Autodesk Inventor part; units mm, degrees
ref_plane "YZ Plane" through (0, 0, 0) normal (1, 0, 0) x (0, 1, 0)
ref_plane "XZ Plane" through (0, 0, 0) normal (0, 1, 0) x (-1, 0, 0)
ref_plane "XY Plane" through (0, 0, 0) normal (0, 0, 1) x (1, 0, 0)
sketch "Sketch2" plane through (0, 0, 0) normal (0, 0, 1) x (1, 0, 0)
  line L0 (0, 12.7) -> (3.6703, 12.7)
  line L1 (0, 12.7) -> (-3.6703, 12.7)
  line L2 (0, 0) -> (3.6703, 0)
  line L3 (0, 0) -> (-3.6703, 0)
  line L4 (-3.6703, 0) -> (-7.3406, 6.35)
  line L5 (-7.3406, 6.35) -> (-3.6703, 12.7)
  line L6 (3.6703, 12.7) -> (7.3406, 6.35)
  line L7 (7.3406, 6.35) -> (3.6703, 0)
  line L8 (0, 0) -> (0, 6.35)
  circle A0 centre (0, 6.35) radius 8.255
  dimension "d11" = 6.35
  dimension "d12" = 16.51
extrude "Extrusion2" add sketch "Sketch2" along normal blind 6.223
sketch "Sketch3" plane through (0, 6.35, 6.223) normal (0, 0, 1) x (1, 0, 0)
  line L0 (-3.6703, -6.35) -> (-7.3406, 0)
  line L1 (-7.3406, 0) -> (-3.6703, 6.35)
  line L2 (-3.6703, 6.35) -> (3.6703, 6.35)
  line L3 (3.6703, 6.35) -> (7.3406, 0)
  line L4 (7.3406, 0) -> (3.6703, -6.35)
  line L5 (3.6703, -6.35) -> (-3.6703, -6.35)
  circle A0 centre (0, 0) radius 8.255
  point P0 (0, -6.35)
extrude "Extrusion3" add sketch "Sketch3" along normal blind 3.302
sketch "Sketch4" plane through (0, 6.35, 9.525) normal (0, 0, 1) x (1, 0, 0)
  line L0 (-7.3406, 0) -> (-3.6703, 6.35)
  line L1 (-3.6703, 6.35) -> (3.6703, 6.35)
  line L2 (3.6703, 6.35) -> (7.3406, 0)
  line L3 (7.3406, 0) -> (3.6703, -6.35)
  line L4 (3.6703, -6.35) -> (-3.6703, -6.35)
  line L5 (-3.6703, -6.35) -> (-7.3406, 0)
  circle A0 centre (0, 0) radius 8.255
  point P0 (0, -6.35)
extrude "Extrusion4" add sketch "Sketch4" along normal blind 6.5786
sketch "Sketch5" plane through (0, 6.35, 16.1036) normal (0, 0, 1) x (1, 0, 0)
  line L0 (-16.3467, 15.7745) -> (15.1254, 15.7745)
  line L1 (15.1254, 15.7745) -> (15.1254, -12.8793)
  line L2 (15.1254, -12.8793) -> (-16.3467, -12.8793)
  line L3 (-16.3467, -12.8793) -> (-16.3467, 15.7745)
  point P0 (0, -6.35)
extrude "Extrusion5" cut sketch "Sketch5" against normal blind 6.5786
sketch "Sketch8" plane through (0, 6.35, 9.525) normal (0, 0, 1) x (1, 0, 0)
  line L0 (-7.3406, 0) -> (-3.6703, -6.35)
  line L1 (-3.6703, 6.35) -> (-7.3406, 0)
  line L2 (3.6703, 6.35) -> (-3.6703, 6.35)
  line L3 (7.3406, 0) -> (3.6703, 6.35)
  line L4 (3.6703, -6.35) -> (7.3406, 0)
  line L5 (-3.6703, -6.35) -> (3.6703, -6.35)
  circle A0 centre (0, 0) radius 8.255
  point P0 (0, -6.35)
extrude "Extrusion7" add sketch "Sketch8" along normal blind 15.875
sketch "Sketch9" plane through (0, 6.35, 25.4) normal (0, 0, 1) x (1, 0, 0)
  line L0 (-7.3406, 0) -> (-3.6703, 6.35)
  line L1 (-3.6703, 6.35) -> (3.6703, 6.35)
  line L2 (3.6703, 6.35) -> (7.3406, 0)
  line L3 (7.3406, 0) -> (3.6703, -6.35)
  line L4 (3.6703, -6.35) -> (-3.6703, -6.35)
  line L5 (-3.6703, -6.35) -> (-7.3406, 0)
  circle A0 centre (0, 0) radius 8.255
  point P0 (0, -6.35)
extrude "Extrusion8" cut sketch "Sketch9" against normal blind 21.7424
sketch "Sketch10" plane through (0, 6.35, 3.6576) normal (0, 0, 1) x (1, 0, 0)
  line L0 (-7.3406, 0) -> (-3.6703, -6.35)
  line L1 (-3.6703, 6.35) -> (-7.3406, 0)
  line L2 (3.6703, 6.35) -> (-3.6703, 6.35)
  line L3 (7.3406, 0) -> (3.6703, 6.35)
  line L4 (3.6703, -6.35) -> (7.3406, 0)
  line L5 (-3.6703, -6.35) -> (3.6703, -6.35)
  circle A0 centre (0, 0) radius 8.255
  point P0 (0, -6.35)
extrude "Extrusion9" add sketch "Sketch10" along normal blind 9.1948
properties part number ".506Spacer"
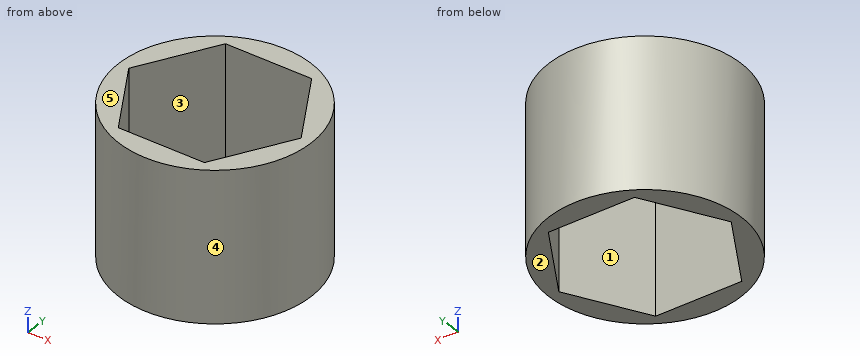
Design review of the part built by this model. Coordinates are the model's own, in mm. Face numbers are marked on the shaded views. A direction names the side the tool comes from. Coordinates: 2 decimals unless noted, no trailing zeros. Write each loop counter-clockwise with the first axis right and the second up, starting at its lowest first coordinate (ties: lowest second). Pieces come first, ordered by that corner, then holes. Notation, with made-up numbers: (50.25, 28.5) - (90.25, 28.5) arc R12 ccw to (90.25, 49.5) - close; hole circle Ø8 at (43, 30.5). An arc over 180 degrees is marked (long way). One line per item, written item: value.
1) For the marked faces 1 and 2, list the 3-axis set-ups (+Z, -Z, +X, -X, +Y, -Y) from which the entire face can be reached by the end or side of a thin tool; tool diameter is ignored.
Answer sheet:
face 1: +Z, -Z
face 2: -Z, +X, -X, +Y, -Y
2) Add section C-C (y = 5). State the section outline as (x, z) points, plus the area to 3 significant figures.
Answer sheet:
outline: (-8.14, 0) - (-6.56, 0) - (-6.56, 12.85) - (-8.14, 12.85) - close; (6.56, 0) - (8.14, 0) - (8.14, 12.85) - (6.56, 12.85) - close
area: 40.7 mm2
3) To check wall thickness, follow probe 1 along Y at (x, z) = (0, 3) (3 decimals); probe 2 along X at (y, z) = (10, 7.25); probe 3 along X at (y, z) = (4.75, 2.5). State the ranges of each line that lie inside material, in increasing order.
Answer sheet:
probe 1: y = -1.905 to 0, 12.7 to 14.605
probe 2: x = -7.4 to -5.23, 5.23 to 7.4
probe 3: x = -8.1 to -6.42, 6.42 to 8.1
4) Add section D-D (y = -0.5). State the section outline as (x, z) points, plus the area to 3 significant figures.
Answer sheet:
outline: (-4.61, 0) - (4.61, 0) - (4.61, 12.85) - (-4.61, 12.85) - close
area: 118 mm2
5) Add section A-A (x = 0). State the section outline as (y, z) points (3 decimals).
Answer sheet:
outline: (-1.905, 0) - (0, 0) - (0, 12.852) - (-1.905, 12.852) - close; (12.7, 0) - (14.605, 0) - (14.605, 12.852) - (12.7, 12.852) - close
6) Add section B-B (z = 7). State the section outline as (x, y) points (3 decimals).
Answer sheet:
outline: circle Ø16.51 at (0, 6.35); hole (-7.341, 6.35) - (-3.67, 0) - (3.67, 0) - (7.341, 6.35) - (3.67, 12.7) - (-3.67, 12.7) - close
7) Mouldability with a two-part tool opening along Y and no side actions: class the marked faces 3, 4 and 5 as +Y half, -Y half, draft (parallel to the pull), parting line (faces both ways), or undercut.
Answer sheet:
face 3: undercut
face 4: parting line
face 5: draft
